```python
from build123d import *

# Parameters (mm, degrees)
SKETCH1_R               = 25.4
SKETCH1_R_2             = 12.7254
BOSS_EXTRUDE1_DEPTH     = 76.2
SKETCH3_R               = 31.75
SKETCH3_R_2             = 12.7254
BOSS_EXTRUDE2_DEPTH     = 12.7
CUT_EXTRUDE3_REACH      = 90.445
CUT_EXTRUDE3_END_RADIUS = 25.4
SKETCH2_R               = 12.7
SKETCH5_W               = 50.8
SKETCH5_H               = 50.8
CUT_EXTRUDE4_DEPTH      = 10.16
SKETCH7_R               = 2.665
CUT_EXTRUDE6_DEPTH      = 6.35
SKETCH8_R               = 2.5
CUT_EXTRUDE7_DEPTH      = 6.35


with BuildPart() as part:
    # Sketch1 → Boss-Extrude1 (new body)
    with BuildSketch(Plane.XY):
        with Locations(Location((0, 0, 0), (0, 0, 180))):
            Circle(SKETCH1_R)
        with Locations(Location((0, 0, 0), (0, 0, 180))):
            Circle(SKETCH1_R_2, mode=Mode.SUBTRACT)
    extrude(amount=BOSS_EXTRUDE1_DEPTH)

    # Sketch3 → Boss-Extrude2 (add)
    with BuildSketch(Plane(origin=(0, 0, 0), x_dir=(-1, 0, 0), z_dir=(0, 0, -1))):
        Circle(SKETCH3_R)
        Circle(SKETCH3_R_2, mode=Mode.SUBTRACT)
    extrude(amount=-BOSS_EXTRUDE2_DEPTH)

    # Cut-Extrude3: up to this cylinder (the profile starts inside it)
    cut_extrude3_end = Plane(origin=(0, 0, 38.1), z_dir=(0, 0, -1)) * Cylinder(CUT_EXTRUDE3_END_RADIUS, 232.69, mode=Mode.PRIVATE)
    # Sketch2 → Cut-Extrude3 (cut, up to the surface)
    with BuildSketch(Plane(origin=(0, 0, 0), x_dir=(1, 0, 0), z_dir=(0, 1, 0)), mode=Mode.PRIVATE) as cut_extrude3_sk1:
        with Locations(Location((0, -38.1, 0), (0, 0, 90))):
            Circle(SKETCH2_R)
    cut_extrude3_tool1 = extrude(cut_extrude3_sk1.sketch, amount=CUT_EXTRUDE3_REACH, mode=Mode.PRIVATE) & cut_extrude3_end
    add(cut_extrude3_tool1.solids().sort_by_distance((0, 0, 38.1))[0], mode=Mode.SUBTRACT)

    # Sketch5 → Cut-Extrude4 (cut)
    with BuildSketch(Plane(origin=(0, 25.4, 0), x_dir=(1, 0, 0), z_dir=(0, 1, 0))):
        with Locations((0, -38.1)):
            Rectangle(SKETCH5_W, SKETCH5_H)
    extrude(amount=-CUT_EXTRUDE4_DEPTH, mode=Mode.SUBTRACT)

    # Sketch7 → Cut-Extrude6 (cut)
    with BuildSketch(Plane(origin=(0, 0, 0), x_dir=(-1, 0, 0), z_dir=(0, 0, -1))):
        with Locations((0, 25.4)):
            Circle(SKETCH7_R)
        with Locations((21.997045256, 12.7)):
            Circle(SKETCH7_R)
        with Locations((21.997045256, -12.7)):
            Circle(SKETCH7_R)
        with Locations((0, -25.4)):
            Circle(SKETCH7_R)
        with Locations((-21.997045256, -12.7)):
            Circle(SKETCH7_R)
        with Locations((-21.997045256, 12.7)):
            Circle(SKETCH7_R)
    extrude(amount=-CUT_EXTRUDE6_DEPTH, mode=Mode.SUBTRACT)

    # Sketch8 → Cut-Extrude7 (cut)
    with BuildSketch(Plane(origin=(0, 15.24, 0), x_dir=(1, 0, 0), z_dir=(0, 1, 0))):
        with Locations(Location((-15.32, -17.7, 0), (0, 0, 270))):
            Circle(SKETCH8_R)
        with Locations(Location((15.32, -17.7, 0), (0, 0, 90))):
            Circle(SKETCH8_R)
        with Locations(Location((-15.32, -58.5, 0), (0, 0, 90))):
            Circle(SKETCH8_R)
        with Locations(Location((15.32, -58.5, 0), (0, 0, 270))):
            Circle(SKETCH8_R)
    extrude(amount=-CUT_EXTRUDE7_DEPTH, mode=Mode.SUBTRACT)


solid = part.part
```
For this review, take the finished solid that the model builds, in its own axes (mm). A direction names the side the tool comes from. Give positions to 0.01 mm unless a question says otherwise; leave off trailing zeros. Order: outer loops, then holes, each group sorted by start corner. A loop starts at its lowest first (then second) coordinate and runs counter-clockwise, first axis right, second up.
1) Take a section at B-B (x = 11). Give the boundary of the cut face in (y, z), then the cut area to 3 significant figures.
2) Take a section at A-A (z = 58.5). Give the boundary of the cut face in (x, y).
3) The part is to be moulded in two halves that separate along Y. For faces 1 (the face through (0, 25, 6.35)), 2 (the face through (6.883, -30.995, 6.261)), 3 (the face through (15, 8.89, 58)), say which applies: released by +Y, released by -Y, zero draft, split by the parting line, or undercut.
4) Take a section at C-C (y = -11). Give the boundary of the cut face in (x, z).
5) For faces 4 (the face through (3.307, -25.184, 44.006)), 5 (the face through (-14, 0, 0)), 6 (the face through (13, 15.24, 38)), 7 (the face through (0.58, 22.8, 3.13)), 8 (the face through (-17.76, 12.11, 17.16)), list the 3-axis set-ups (+Z, -Z, +X, -X, +Y, -Y) from which the entire face can be reached by the end or side of a thin tool; tool diameter is ignored.
6) Wall thickness on line 1 (Z direction, x = 15, y = 12); line 2 (Y direction, x = 0, z = 3) (3 decimals); line 3 (Y direction, x = 0, z = 7.5): over which ranges is each line inside the solid? List them lowest first.
7) Insertion check: pin 1 (10 mm diameter, centred on x = -2, y = 5.5, fed in from +Z); pin 2 (6 mm diameter, centred on y = 4.5, z = 63, fed in from +X); pin 3 (6 mm diameter, centred on x = -15.32, z = 17.7, fed in from +Y); pin 4 (1 mm diameter, centred on y = 13, z = 59.5, fed in from +X). Each pin has a flat end and moves straight along its axis. Give the tip position at first contact, or say it passes through.
8) Take a section at D-D (z = 38.1). Give the boundary of the cut face in (x, y).
Derived:
1. outline: (-29.78, 0) - (-6.4, 0) - (-6.4, 76.2) - (-22.89, 76.2) - (-22.89, 12.7) - (-29.78, 12.7) - close; (6.4, 0) - (29.78, 0) - (29.78, 12.7) - (15.24, 12.7) - (15.24, 31.75) - (6.4, 31.75) - close; (6.4, 44.45) - (15.24, 44.45) - (15.24, 63.5) - (22.89, 63.5) - (22.89, 76.2) - (6.4, 76.2) - close
1. area: 2,190 mm2
2. outline: (-20.32, 15.24) arc R25.4 ccw (long way) to (20.32, 15.24) - (17.82, 15.24) - (17.82, 8.89) - (12.82, 8.89) - (12.82, 15.24) - (-12.82, 15.24) - (-12.82, 8.89) - (-17.82, 8.89) - (-17.82, 15.24) - close; hole circle Ø25.45 at (0, 0)
3. face 1: undercut
3. face 2: split by the parting line
3. face 3: released by +Y
4. outline: (-29.78, 0) - (-24.05, 0) - (-24.05, 6.35) - (-19.94, 6.35) - (-19.94, 0) - (-6.4, 0) - (-6.4, 76.2) - (-22.89, 76.2) - (-22.89, 12.7) - (-29.78, 12.7) - close; (6.4, 0) - (19.94, 0) - (19.94, 6.35) - (24.05, 6.35) - (24.05, 0) - (29.78, 0) - (29.78, 12.7) - (22.89, 12.7) - (22.89, 76.2) - (6.4, 76.2) - close
5. face 4: +Z
5. face 5: -Z, +X, -X, +Y, -Y
5. face 6: +X, -X, +Y
5. face 7: -Z
5. face 8: +Y
6. line 1: z = 0 to 15.22, 20.18 to 56.02, 60.98 to 76.2
6. line 2: y = -31.75 to -28.065, -22.735 to -12.725, 12.725 to 22.735, 28.065 to 31.75
6. line 3: y = -31.75 to -12.73, 12.73 to 31.75
7. pin 1: passes through
7. pin 2: stops at x = 25.36
7. pin 3: stops at y = 15.24
7. pin 4: stops at x = 22.11
8. outline: (-20.32, 15.24) arc R25.4 ccw (long way) to (20.32, 15.24) - (12.7, 15.24) - (12.7, 0.8) arc R12.73 cw (long way) to (-12.7, 0.8) - (-12.7, 15.24) - close
